```python
from build123d import *

# Parameters (mm, degrees)
SKETCH1_R           = 22
SKETCH1_R_2         = 1.5
SKETCH1_W           = 20
SKETCH1_H           = 20
BOSS_EXTRUDE1_DEPTH = 3


with BuildPart() as part:
    # Sketch1 → Boss-Extrude1 (new body)
    with BuildSketch(Plane(origin=(0, 0, 0), x_dir=(1, 0, 0), z_dir=(0, 1, 0))):
        Circle(SKETCH1_R)
        with Locations((-15, 0)):
            Circle(SKETCH1_R_2, mode=Mode.SUBTRACT)
        with Locations((0, 15)):
            Circle(SKETCH1_R_2, mode=Mode.SUBTRACT)
        with Locations((15, 0)):
            Circle(SKETCH1_R_2, mode=Mode.SUBTRACT)
        with Locations((0, -15)):
            Circle(SKETCH1_R_2, mode=Mode.SUBTRACT)
        Rectangle(SKETCH1_W, SKETCH1_H, mode=Mode.SUBTRACT)
    extrude(amount=BOSS_EXTRUDE1_DEPTH)


solid = part.part
```
Input: part model. Units: mm. Frame: model coordinates. Round coordinates to 2 decimals unless told otherwise and drop trailing zeros. Loops run counter-clockwise (first coordinate to the right, second up) from the corner with the lowest first, then second, coordinate; pieces in that order, holes last. Notation, with made-up numbers: (87.5, 65) -> (127.5, 65) arc R26 ccw to (127.5, 80) -> close; hole circle Ø7 at (44.5, 41.5). An arc over 180 degrees is marked (long way). One line per item, written item: value.
(1) Section A-A (x = -9). Return the cut outline in (y, z).
Geometry check:
outline: (0, -20.07) -> (3, -20.07) -> (3, -10) -> (0, -10) -> close; (0, 10) -> (3, 10) -> (3, 20.07) -> (0, 20.07) -> close
(2) Pin query (flat end, axial travel): pin 1 (1 mm diameter, centred on x = 9.5, y = 2, fed in from -Z); pin 2 (0.9 mm diameter, centred on y = 1.5, z = 2, fed in from -X); pin 3 (3 mm diameter, centred on x = -6, z = 16, fed in from -Y); pin 4 (1.5 mm diameter, centred on y = 1.5, z = -15, fed in from -X). Return the tip coordinate at first contact, or that it passes through.
Geometry check:
pin 1: z = -20.07
pin 2: x = -21.95
pin 3: y = 0
pin 4: x = -16.76
(3) Section B-B (z = 0). Return the cut outline in (x, y), plus the area to 3 significant figures.
Geometry check:
outline: (-22, 0) -> (-16.5, 0) -> (-16.5, 3) -> (-22, 3) -> close; (-13.5, 0) -> (-10, 0) -> (-10, 3) -> (-13.5, 3) -> close; (10, 0) -> (13.5, 0) -> (13.5, 3) -> (10, 3) -> close; (16.5, 0) -> (22, 0) -> (22, 3) -> (16.5, 3) -> close
area: 54.0 mm2
(4) Section C-C (y = 1.5). Return the cut outline in (x, z).
Geometry check:
outline: circle Ø44 at (0, 0); hole circle Ø3 at (-15, 0); hole (-10, -10) -> (10, -10) -> (10, 10) -> (-10, 10) -> close; hole circle Ø3 at (0, -15); hole circle Ø3 at (0, 15); hole circle Ø3 at (15, 0)
(5) Section D-D (z = 9). Return the cut outline in (x, y).
Geometry check:
outline: (-20.07, 0) -> (-10, 0) -> (-10, 3) -> (-20.07, 3) -> close; (10, 0) -> (20.07, 0) -> (20.07, 3) -> (10, 3) -> close
(6) Mould query, pull axis Z, two halves, no side actions, for faces 1 (the face through (-16.5, 1.48, -0.07)), 2 (the face through (-4.769, 1.479, 21.477)). Classes: pulls with the +Z half, pulls with the -Z half, needs draft (parallel to the pull), parting line crosses it, or undercut.
Geometry check:
face 1: undercut
face 2: parting line crosses it
(7) Material intervals for line 1 (X direction, y = 2, z = 0); line 2 (Z direction, x = -1, y = 1.55), sorted ascending. Write a range as [from, to].
Geometry check:
line 1: [-22, -16.5], [-13.5, -10], [10, 13.5], [16.5, 22]
line 2: [-21.98, -16.12], [-13.88, -10], [10, 13.88], [16.12, 21.98]
